from build123d import *

# Parameters (mm, degrees)
BOSS_EXTRUDE1_DEPTH  = 19.05
FILLET1_R            = 30
FILLET2_R            = 20
BOSS_EXTRUDE3_DEPTH  = 19.05
SKETCH14_W           = 12
SKETCH14_H           = 10
CUT_EXTRUDE1_DEPTH   = 39
CUT_SWEEP1_PROFILE_R = 6.35
SKETCH24_W           = 5
SKETCH24_H           = 15
SKETCH24_W_2         = 15
SKETCH24_H_2         = 5
CUT_EXTRUDE2_DEPTH   = 10


with BuildPart() as part:
    # Sketch1 → Boss-Extrude1 (new body)
    with BuildSketch(Plane.XY):
        Polygon((-100, 0), (0, 0), (0, 250), (65, 250), (65, 211.9), (38.1, 211.9), (38.1, -38.1), (-100, -38.1), align=None)
    extrude(amount=BOSS_EXTRUDE1_DEPTH)

    # Fillet1
    fillet1_edges = [part.edges().sort_by_distance(p)[0] for p in [
        (0, 250, 9.525),
        (38.1, -38.1, 9.525),
    ]]
    fillet(fillet1_edges, radius=FILLET1_R)

    # Fillet2
    fillet2_edges = [part.edges().sort_by_distance(p)[0] for p in [
        (0, 0, 9.525),
    ]]
    fillet(fillet2_edges, radius=FILLET2_R)

    # Sketch13 → Boss-Extrude3 (add)
    with BuildSketch(Plane.XY.offset(19.05)):
        Polygon((55, 221.425), (43, 221.425), (43, 211.425), (51, 211.425), (51, 189.425), (41, 189.425), (41, 171.425), (36.549895251, 171.425), (36.549895251, 223.572995821), (65, 223.572995821), (65, 211.9), (65, 211.425), (55, 211.425), align=None)
    extrude(amount=-BOSS_EXTRUDE3_DEPTH)

    # Sketch14 → Cut-Extrude1 (cut)
    with BuildSketch(Plane.XY.offset(19.05)):
        with Locations((49, 216.42)):
            Rectangle(SKETCH14_W, SKETCH14_H)
    extrude(amount=-CUT_EXTRUDE1_DEPTH, mode=Mode.SUBTRACT)

    # Cut-Sweep1: sweep along a path in Sketch17
    with BuildLine(Plane.XY.offset(19.05)) as cut_sweep1_path:
        Line((65, 230.95), (39.05, 230.95))
        ThreePointArc((39.05, 230.95), (24.907864376, 225.092135624), (19.05, 210.95))
        Line((19.05, 210.95), (19.05, 0.95))
        ThreePointArc((19.05, 0.95), (13.192135624, -13.192135624), (-0.95, -19.05))
        Line((-0.95, -19.05), (-100, -19.05))
    # Cut-Sweep1 profile (on start of the path) → Cut-Sweep1 (sweep, cut)
    with BuildSketch(Plane(origin=(65, 230.95, 19.05), x_dir=(0, 0, -1), z_dir=(-1, 0, 0))):
        Circle(CUT_SWEEP1_PROFILE_R)
    sweep(path=cut_sweep1_path.line, mode=Mode.SUBTRACT)

    # Sketch24 → Cut-Extrude2 (cut)
    with BuildSketch(Plane.XY.offset(19.05)):
        with Locations((6.35, 120)):
            Rectangle(SKETCH24_W, SKETCH24_H)
        with Locations((-60, -6.35)):
            Rectangle(SKETCH24_W_2, SKETCH24_H_2)
        with Locations((31.75, 120)):
            Rectangle(SKETCH24_W, SKETCH24_H)
        with Locations((-60, -31.75)):
            Rectangle(SKETCH24_W_2, SKETCH24_H_2)
    extrude(amount=-CUT_EXTRUDE2_DEPTH, mode=Mode.SUBTRACT)


solid = part.part
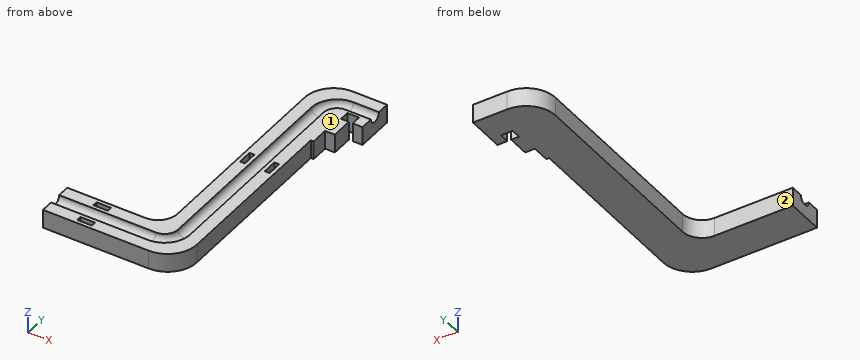
Verification items for the finished model (mm, model axes). Face numbers are marked on the shaded views. A direction names the side the tool comes from. Coordinates: 2 decimals unless noted, no trailing zeros. Write each loop counter-clockwise with the first axis right and the second up, starting at its lowest first coordinate (ties: lowest second). Pieces come first, ordered by that corner, then holes. Notation, with made-up numbers: (-3.5, -32) - (22.5, -32) arc R13 ccw to (22.5, -27) - close; hole circle Ø7 at (-3, 1.25). An arc over 180 degrees is marked (long way). Answer as a JSON object with one key per item and string values.
(1) Cross-section at C-C on x = -81. Record the cut outline in (y, z).
Report:
{"outline": "(-38.1, 0) - (0, 0) - (0, 19.05) - (-12.7, 19.05) arc R6.35 cw to (-25.4, 19.05) - (-38.1, 19.05) - close"}
(2) Gauge pin test, flat ends, axial feed: pin 1 Ø5 at (x, z) = (-61, 15.5) entering from +Y; pin 2 Ø3 at (x, z) = (48, 7) entering from -Y (3 decimals); pin 3 Ø2 at (y, z) = (28.5, 15.5) entering from +X. Record the tip position at first contact, or that the pin passes through.
Report:
{"pin 1": "y = 0", "pin 2": "y = 189.425", "pin 3": "x = 38.1"}
(3) Thickness scan on line 1 along Y through (x, z) = (-66.5, 12); line 2 along Y through (x, z) = (49.5, 10.75) (3 decimals); line 3 along X through (y, z) = (219, 3). Record the ranges inside material, lowest first.
Report:
{"line 1": "-38.1 to -34.25, -29.25 to -8.85, -3.85 to 0", "line 2": "189.425 to 211.42, 221.42 to 250", "line 3": "0 to 43, 55 to 65"}
(4) Cross-section at B-B on z = 5.75. Record the cut outline in (x, y) (3 decimals).
Report:
{"outline": "(-100, -38.1) - (8.1, -38.1) arc R30 ccw to (38.1, -8.1) - (38.1, 171.425) - (41, 171.425) - (41, 189.425) - (51, 189.425) - (51, 211.42) - (43, 211.42) - (43, 221.42) - (55, 221.42) - (55, 211.425) - (65, 211.425) - (65, 250) - (30, 250) arc R30 ccw to (0, 220) - (0, 20) arc R20 cw to (-20, 0) - (-100, 0) - close"}
(5) Tool access check on the marked faces 1 and 2. Record the directions out of +Z, -Z, +X, -X, +Y, -Y that give a thin tool (end or side, any length) a straight path to the whole face; none if there is none.
Report:
{"face 1": "+Z, +X, -X, +Y, -Y", "face 2": "+Z, -Z, -X, +Y"}
(6) Cross-section at A-A on y = 44. Record the cut outline in (x, z), plus the area to 3 significant figures.
Report:
{"outline": "(0, 0) - (38.1, 0) - (38.1, 19.05) - (25.4, 19.05) arc R6.35 cw to (12.7, 19.05) - (0, 19.05) - close", "area": "662 mm^2"}
